Design review of the part built by this model. Coordinates are the model's own, in mm. A direction names the side the tool comes from. Coordinates: 2 decimals unless noted, no trailing zeros. Write each loop counter-clockwise with the first axis right and the second up, starting at its lowest first coordinate (ties: lowest second). Pieces come first, ordered by that corner, then holes. Notation, with made-up numbers: (46.5, 49.25) -> (79.5, 49.25) arc R21 cw to (79.5, 73.25) -> close; hole circle Ø9 at (42.5, 31.25). An arc over 180 degrees is marked (long way). Answer in a Markdown table with one row per item. Add a question column.
Item 1: Draft analysis for pull direction Z (two halves, no side actions). For faces 1 (the face through (23.4, 37.06, 17.26)), 2 (the face through (57.535, -3.252, 5.357)), 3 (the face through (60, -20, 20)), 4 (the face through (55, 0, 20)), state which applies: released by +Z, released by -Z, zero draft, split by the parting line, or undercut.
Item 2: Take a section at A-A, the plane x = 5. Write out the cut boundary in (y, z).
Item 3: Clearance check with flat-ended pins moving along their axes: P1, Ø2, axis at x = 47, z = 12.5, coming from the +Y side; P2, Ø15, axis at y = 1.5, z = 15, coming from the +X side. State where each tip first meets the part, or that it passes through.
Item 4: Take a section at B-B, the plane z = 20. Write out the cut boundary in (x, y).
Item 5: For faces 5 (the face through (37.37, 33.19, 26.76)), 6 (the face through (59, 0, 38)), list the 3-axis set-ups (+Z, -Z, +X, -X, +Y, -Y) from which the entire face can be reached by the end or side of a thin tool; tool diameter is ignored.
Item 6: To check wall thickness, follow line 1 (Y direction, x = 30, z = 30.5); line 2 (Y direction, x = 56.4, z = 20); line 3 (Y direction, x = 58.5, z = 20). State the ranges of each line that lie inside material, in increasing order.
Item 7: Take a section at C-C, the plane x = 30. Write out the cut boundary in (y, z), and give its area (3 significant figures).
Item 8: Take a section at D-D, the plane z = 33.5. Write out the cut boundary in (x, y), and give its area (3 significant figures).
from build123d import *

# Parameters (mm, degrees)
F0_W     = 120
F0_H     = 65
F1_DEPTH = 40
F2_R     = 5
F3_R     = 15
F4_DEPTH = 5
F5_R     = 10
F6_DEPTH = 5
F7_SIZE  = 3


with BuildPart() as f1:
    # F0 (on Top) → F1 (new body)
    with BuildSketch(Plane.XY):
        with Locations((0, -0.295118)):
            Rectangle(F0_W, F0_H)
    extrude(amount=F1_DEPTH)

    # F2
    f2_edges = [f1.edges().sort_by_distance(p)[0] for p in [
        (-60, -32.795118, 20),
        (60, -32.795118, 20),
        (60, 32.204882, 20),
        (-60, 32.204882, 20),
        (0, 32.204882, 40),
        (60, -0.295118, 40),
        (0, -32.795118, 40),
        (-60, -0.295118, 40),
        (0, 32.204882, 0),
        (0, -32.795118, 0),
        (-60, -0.295118, 0),
        (60, -0.295118, 0),
    ]]
    fillet(f2_edges, radius=F2_R)

    # F3 (on face) → F4 (cut)
    with BuildSketch(Plane.YZ.offset(60)):
        with Locations((0, 20)):
            Circle(F3_R)
    extrude(amount=-F4_DEPTH, mode=Mode.SUBTRACT)

    # F5 (on face) → F6 (join)
    with BuildSketch(Plane(origin=(0, 32.204882, 0), x_dir=(-1, 0, 0), z_dir=(0, 1, 0))):
        with Locations((-30, 20)):
            Circle(F5_R)
    extrude(amount=F6_DEPTH)

    # F7
    f7_edges = [f1.edges().sort_by_distance(p)[0] for p in [
        (40, 37.204882, 20),
    ]]
    chamfer(f7_edges, length=F7_SIZE)


solid = f1.part
Answers:
| question | item | result |
|---|---|---|
| 1 | face 1 | split by the parting line |
| 1 | face 2 | undercut |
| 1 | face 3 | zero draft |
| 1 | face 4 | undercut |
| 2 | outline | (-32.8, 5) arc R5 ccw to (-27.8, 0) -> (27.2, 0) arc R5 ccw to (32.2, 5) -> (32.2, 35) arc R5 ccw to (27.2, 40) -> (-27.8, 40) arc R5 ccw to (-32.8, 35) -> close |
| 3 | P1 | stops at y = 32.2 |
| 3 | P2 | stops at x = 55 |
| 4 | outline | (-60, -27.8) arc R5 ccw to (-55, -32.8) -> (55, -32.8) arc R5 ccw to (60, -27.8) -> (60, -15) -> (55, -15) -> (55, 15) -> (60, 15) -> (60, 27.2) arc R5 ccw to (55, 32.2) -> (40, 32.2) -> (40, 34.2) -> (37, 37.2) -> (23, 37.2) -> (20, 34.2) -> (20, 32.2) -> (-55, 32.2) arc R5 ccw to (-60, 27.2) -> close |
| 5 | face 5 | +Y |
| 5 | face 6 | +Z, +X, +Y, -Y |
| 6 | line 1 | y = -32.8 to 32.2 |
| 6 | line 2 | y = -32.6 to -15, 15 to 32 |
| 6 | line 3 | y = -31.37 to -15, 15 to 30.78 |
| 7 | outline | (-32.8, 5) arc R5 ccw to (-27.8, 0) -> (27.2, 0) arc R5 ccw to (32.2, 5) -> (32.2, 10) -> (34.2, 10) -> (37.2, 13) -> (37.2, 27) -> (34.2, 30) -> (32.2, 30) -> (32.2, 35) arc R5 ccw to (27.2, 40) -> (-27.8, 40) arc R5 ccw to (-32.8, 35) -> close |
| 7 | area | 2,670 mm^2 |
| 8 | outline | (-60, -27.8) arc R5 ccw to (-55, -32.8) -> (55, -32.8) arc R5 ccw to (60, -27.8) -> (60, -6.54) -> (55, -6.54) -> (55, 6.54) -> (60, 6.54) -> (60, 27.2) arc R5 ccw to (55, 32.2) -> (-55, 32.2) arc R5 ccw to (-60, 27.2) -> close |
| 8 | area | 7,710 mm^2 |
